Autodesk Inventor part; units mm, degrees
ref_plane "YZ Plane" through (0, 0, 0) normal (1, 0, 0) x (0, 1, 0)
ref_plane "XZ Plane" through (0, 0, 0) normal (0, 1, 0) x (-1, 0, 0)
ref_plane "XY Plane" through (0, 0, 0) normal (0, 0, 1) x (1, 0, 0)
sketch "Sketch1" plane through (0, 0, 0) normal (0, 1, 0) x (-1, 0, 0)
  circle A0 centre (0, 0) radius 3.175
  dimension "d0" = 6.35
extrude "Extrusion1" add sketch "Sketch1" along normal blind 101.6
sketch "Sketch2" plane through (0, 101.6, 0) normal (0, 1, 0) x (1, 0, 0)
  line L0 (6.35, -15.748) -> (-6.35, -15.748)
  line L1 (-6.35, -15.748) -> (-6.35, 15.748)
  line L2 (-6.35, 15.748) -> (6.35, 15.748)
  line L3 (6.35, 15.748) -> (6.35, -15.748)
  line L4 (6.35, -15.748) -> (-6.35, 15.748) construction
  line L5 (-6.35, -15.748) -> (6.35, 15.748) construction
  point P0 (0, 0)
  dimension "d3" = 12.7
  dimension "d4" = 31.496
extrude "Extrusion2" add sketch "Sketch2" along normal blind 3.175
sketch "Sketch3" plane through (0, 104.775, 0) normal (0, 1, 0) x (1, 0, 0)
  point P0 (0, 0)
sketch "Sketch4" plane through (0, 104.775, 0) normal (0, 1, 0) x (1, 0, 0)
  line L0 (6.35, -15.748) -> (6.35, 15.748)
  line L1 (-6.35, -15.748) -> (6.35, -15.748)
  line L2 (6.35, -15.748) -> (6.35, -12.573)
  line L3 (6.35, -12.573) -> (-6.35, -12.573)
  line L4 (-6.35, -12.573) -> (-6.35, -15.748)
  line L5 (-6.35, 15.748) -> (6.35, 15.748)
  line L6 (6.35, 15.748) -> (6.35, 12.573)
  line L7 (6.35, 12.573) -> (-6.35, 12.573)
  line L8 (-6.35, 12.573) -> (-6.35, 15.748)
  line L9 (6.35, 15.748) -> (-6.35, 15.748)
  point P0 (0, 0)
  dimension "d7" = 3.175
  dimension "d8" = 3.175
  dimension "d9" = 0
extrude "Extrusion3" add sketch "Sketch4" along normal blind 15.875
sketch "Sketch5" plane through (6.35, 101.6, -15.748) normal (0, 0, -1) x (-1, 0, 0)
  circle A0 centre (6.35, 12.7) radius 3.175
  line L0 (12.7, 0) -> (0, 0)
  point P0 (6.35, -101.6)
  dimension "d12" = 6.35
  dimension "d13" = 12.7
extrude "Extrusion4" cut sketch "Sketch5" against normal blind 50.8
properties part number "PC3.5-ROD"
Geometry: final body of the model. Coordinates: model frame, mm. A direction names the side the tool comes from. Coordinates: 2 decimals unless noted, no trailing zeros. Order: outer loops, then holes, each group sorted by start corner. A loop starts at its lowest first (then second) coordinate and runs counter-clockwise, first axis right, second up. Notation, with made-up numbers: (36, 15.5) -> (61, 15.5) arc R19 cw to (61, 19.5) -> close; hole circle Ø6 at (41.5, 0). An arc over 180 degrees is marked (long way). Write item = value, one per line.
(1) Cut plane A-A on x = 0. Return loops of the section in (y, z) (3 decimals), plus the area to 3 significant figures.
Solved:
outline = (0, -3.175) -> (101.6, -3.175) -> (101.6, -15.748) -> (111.125, -15.748) -> (111.125, -12.573) -> (104.775, -12.573) -> (104.775, 12.573) -> (111.125, 12.573) -> (111.125, 15.748) -> (101.6, 15.748) -> (101.6, 3.175) -> (0, 3.175) -> close; (117.475, -15.748) -> (120.65, -15.748) -> (120.65, -12.573) -> (117.475, -12.573) -> close; (117.475, 12.573) -> (120.65, 12.573) -> (120.65, 15.748) -> (117.475, 15.748) -> close
area = 806 mm²
(2) Cut plane C-C on z = 0. Return loops of the section in (x, y) (3 decimals).
Solved:
outline = (-6.35, 101.6) -> (-3.175, 101.6) -> (-3.175, 0) -> (3.175, 0) -> (3.175, 101.6) -> (6.35, 101.6) -> (6.35, 104.775) -> (-6.35, 104.775) -> close
(3) Cut plane B-B on y = 107. Return loops of the section in (x, z), plus the area to 3 significant figures.
Solved:
outline = (-6.35, -15.75) -> (6.35, -15.75) -> (6.35, -12.57) -> (-6.35, -12.57) -> close; (-6.35, 12.57) -> (6.35, 12.57) -> (6.35, 15.75) -> (-6.35, 15.75) -> close
area = 80.6 mm²
(4) Cut plane D-D on x = 5. Return loops of the section in (y, z) (3 decimals), plus the area to 3 significant figures.
Solved:
outline = (101.6, -15.748) -> (120.65, -15.748) -> (120.65, -12.573) -> (104.775, -12.573) -> (104.775, 12.573) -> (120.65, 12.573) -> (120.65, 15.748) -> (101.6, 15.748) -> close
area = 201 mm²
(5) Pull-direction query (Z, two-part tool) for faces 3 (the cylindrical face through (0.69, 50.09, 3.1)), 4 (the flat face through (0, 104.775, 0)), 5 (the flat face through (0, 120.65, -14)); classes: pulls with the +Z half, pulls with the -Z half, needs draft (parallel to the pull), parting line crosses it, or undercut.
Solved:
face_3 = parting line crosses it
face_4 = undercut
face_5 = needs draft
(6) Line query: line 1 (Y direction, x = 0, z = -13.5) (3 decimals); line 2 (X direction, y = 114, z = -13); line 3 (Y direction, x = 1.5, z = -5.5) (3 decimals). Output: solid intervals per line, ascending.
Solved:
line_1 = 101.6 to 111.125, 117.475 to 120.65
line_2 = -6.35 to -3.16, 3.16 to 6.35
line_3 = 101.6 to 104.775
(7) Pin query (flat end, axial travel): pin 1 Ø2 at (y, z) = (29.5, 0.5) entering from +X (3 decimals); pin 2 Ø2 at (x, y) = (-2, 54) entering from -Z; pin 3 Ø4 at (x, z) = (2, -6) entering from +Y (3 decimals). Return the tip coordinate at first contact, or that it passes through.
Solved:
pin_1 = 3.175
pin_2 = -3.01
pin_3 = 104.775
(8) Access query for faces 1 (the flat face through (0.1, 110.8, 12.573)), 2 (the cylindrical face through (0.69, 111.2, 14.14)). Directions: +Z, -Z, +X, -X, +Y, -Y. A direction counts if a zero-diameter tool reaches every point of the face in a straight line with its end or side. Return the directions, or none.
Solved:
face_1 = +X, -X, +Y
face_2 = +Z, -Z
